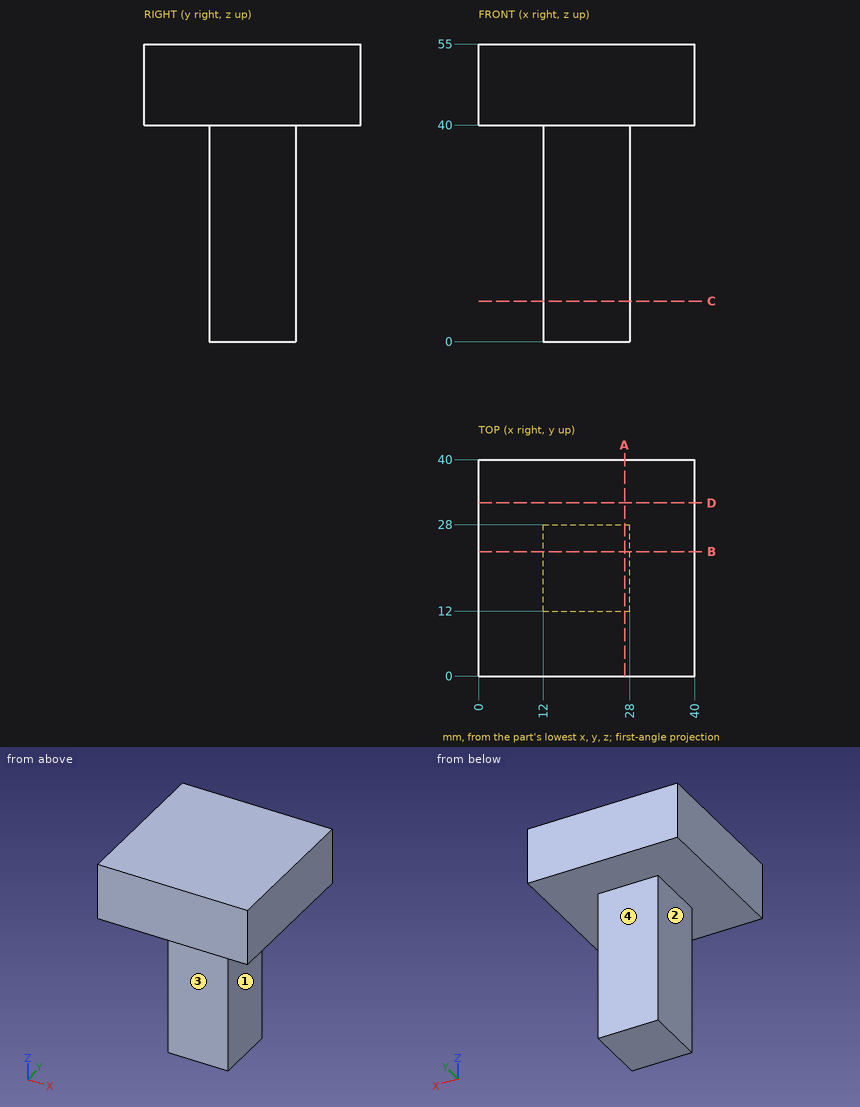
Here's the drawing with two shaded views (mm, measured from the low corner). I have some questions. A direction names the side the tool comes from. Give positions to 0.01 mm unless a question says otherwise; leave off trailing zeros. Loops run counter-clockwise (first coordinate to the right, second up) from the corner with the lowest first, then second, coordinate; pieces in that order, holes last. Notation, with made-up numbers: (49, -22) - (74, -22) arc R25 cw to (74, 9) - close; hole circle Ø7 at (66.25, -18.5). An arc over 180 degrees is marked (long way). One line per item, written item: value.
(1) I'm going to push flat-ended pins straight in: pin 1 (5 mm diameter, centred on y = 26, z = 9.5, fed in from +X); pin 2 (13 mm diameter, centred on y = 16, z = 29, fed in from -X); pin 3 (13 mm diameter, centred on x = 22, z = 21.5, fed in from +Y); pin 4 (5 mm diameter, centred on x = 29.5, z = 46, fed in from -Y). Where does each tip first touch, or does it pass through?
Verdict:
pin 1: x = 28
pin 2: x = 12
pin 3: y = 28
pin 4: y = 0
(2) If we section it at A-A, the plane x = 27: List the corners of the cut face in (y, z) for me, plus the area to 3 significant figures.
Verdict:
outline: (0, 40) - (12, 40) - (12, 0) - (28, 0) - (28, 40) - (40, 40) - (40, 55) - (0, 55) - close
area: 1,240 mm^2
(3) On a 3-axis mill with a long thin cutter (end or side, diameter ignored), from which of +Z, -Z, +X, -X, +Y, -Y can I reach the whole of each face in a straight line? I mean the marked faces 1, 2, 3 and 4. Say none if no direction works.
Verdict:
face 1: -Z, +X, +Y, -Y
face 2: -Z, -X, +Y, -Y
face 3: -Z, +X, -X, -Y
face 4: -Z, +X, -X, +Y
(4) I need wall thicknesses on line 1 along Z through (x, y) = (30, 25.5); line 2 along X through (y, z) = (27, 26). Which ranges of each line are inside material? Lowest first, please.
Verdict:
line 1: 40 to 55
line 2: 12 to 28
(5) If we section it at C-C, the plane z = 7.5: List the corners of the cut face in (x, y) for me, plus the area to 3 significant figures.
Verdict:
outline: (12, 12) - (28, 12) - (28, 28) - (12, 28) - close
area: 256 mm^2
(6) If we section it at D-D, the plane y = 32: List the corners of the cut face in (x, z) for me.
Verdict:
outline: (0, 40) - (40, 40) - (40, 55) - (0, 55) - close
